Read the model definition and answer for the solid it produces. Units are mm, in the model's axes. A direction names the side the tool comes from. Give positions to 0.01 mm unless a question says otherwise; leave off trailing zeros. Order: outer loops, then holes, each group sorted by start corner. A loop starts at its lowest first (then second) coordinate and runs counter-clockwise, first axis right, second up. Notation, with made-up numbers: (47.5, -34) - (65.5, -34) arc R11 ccw to (65.5, -25) - close; hole circle Ø4 at (54.5, -38). An arc over 180 degrees is marked (long way). Write each question's results on one line, items separated by ' | '. Start each with the question number.
Q1. A tool of negligible diameter and unlimited length cuts with its end or side. For faces 4 (the face through (33.718, -21, 88)), 5 (the face through (9, -2, 0)), from which of +Z, -Z, +X, -X, +Y, -Y can it reach the whole face along a straight path? Write none if from no direction.
Q2. Flat-ended cylindrical pins translate along their axes: P1, Ø6, axis at x = -6, y = -4.5, coming from the -Z side; P2, Ø18.5, axis at x = 1, z = 58, coming from the -Y side (3 decimals); P3, Ø3.5, axis at x = -36.5, z = 127.5, coming from the -Y side; P4, Ø1.5, axis at y = -19.5, z = 53, coming from the -X side. Find the tip coordinate at first contact, or state that the pin passes through.
Q3. Find section B-B on x = -6.5. Give the vertices of the cut face in (y, z) (3 decimals), and give its area (3 significant figures).
Q4. Find section C-C on y = -23. Give the vertices of the cut face in (x, z).
Q5. Find section A-A on z = 107. Give the vertices of the cut face in (x, y) (1 decimal).
Q6. For a pull along X with two mould halves and no side action, classify faces 1 (the face through (38.164, -17, 88)), 2 (the face through (-33.718, -10, 88)), 3 (the face through (-36, -12.319, 88)) as +X half, -X half, draft (parallel to the pull), parting line (faces both ways), or undercut.
Q7. Find the intervals of material crossed by line 1 along X through (y, z) = (-9.5, 121); line 2 along Y through (x, z) = (1, 128.5) (3 decimals); line 3 along X through (y, z) = (-16.5, 94), in increasing order. Write a range as from..to.
from build123d import *

# Parameters (mm, degrees)
BOSS_EXTRUDE1_DEPTH = 177.8
FILLET1_R           = 2.54
FILLET2_R           = 2.54


with BuildPart() as part:
    # Sketch1 → Boss-Extrude1 (new body)
    with BuildSketch(Plane.XY):
        Polygon((0, 0), (38.1635, 0), (38.1635, -34.925), (33.7185, -34.925), (33.7185, -4.445), (-33.7185, -4.445), (-33.7185, -12.319), (-38.1635, -12.319), (-38.1635, 0), align=None)
    extrude(amount=BOSS_EXTRUDE1_DEPTH)

    # Fillet1
    fillet1_edges = [part.edges().sort_by_distance(p)[0] for p in [
        (33.7185, -4.445, 88.9),
    ]]
    fillet(fillet1_edges, radius=FILLET1_R)

    # Fillet2
    fillet2_edges = [part.edges().sort_by_distance(p)[0] for p in [
        (-33.7185, -4.445, 88.9),
    ]]
    fillet(fillet2_edges, radius=FILLET2_R)


solid = part.part
Working result:
1) face 4: +Z, -Z, -Y | face 5: -Z, +X, -X, +Y, -Y
2) P1: z = 0 | P2: y = -4.445 | P3: y = -12.32 | P4: x = 33.72
3) outline: (-4.445, 0) - (0, 0) - (0, 177.8) - (-4.445, 177.8) - close | area: 790 mm²
4) outline: (33.72, 0) - (38.16, 0) - (38.16, 177.8) - (33.72, 177.8) - close
5) outline: (-38.2, -12.3) - (-33.7, -12.3) - (-33.7, -7) arc R2.5 cw to (-31.2, -4.4) - (31.2, -4.4) arc R2.5 cw to (33.7, -7) - (33.7, -34.9) - (38.2, -34.9) - (38.2, 0) - (-38.2, 0) - close
6) face 1: +X half | face 2: undercut | face 3: draft
7) line 1: -38.16..-33.72, 33.72..38.16 | line 2: -4.445..0 | line 3: 33.72..38.16
